from build123d import *

# Parameters (mm, degrees)
CROQUIS1_W              = 163
CROQUIS1_H              = 163
SALIENTE_EXTRUIR1_DEPTH = 3.3
CROQUIS2_R              = 5
SALIENTE_EXTRUIR2_DEPTH = 3
REDONDEO1_R             = 1
CROQUIS3_R              = 3.25
CORTAR_EXTRUIR1_DEPTH   = 3
CROQUIS4_R              = 1.75
CORTAR_EXTRUIR2_DEPTH   = 6.3


with BuildPart() as part:
    # Croquis1 → Saliente-Extruir1 (new body)
    with BuildSketch(Plane(origin=(0, 0, 0), x_dir=(1, 0, 0), z_dir=(0, 1, 0))):
        Rectangle(CROQUIS1_W, CROQUIS1_H)
    extrude(amount=-SALIENTE_EXTRUIR1_DEPTH)

    # Croquis2 → Saliente-Extruir2 (add)
    with BuildSketch(Plane(origin=(0, 0, 0), x_dir=(1, 0, 0), z_dir=(0, 1, 0))):
        with Locations((-75.5, 75.5)):
            Circle(CROQUIS2_R)
        with Locations((75.5, 75.5)):
            Circle(CROQUIS2_R)
        with Locations((-75.5, -75.5)):
            Circle(CROQUIS2_R)
        with Locations((75.5, -75.5)):
            Circle(CROQUIS2_R)
    extrude(amount=SALIENTE_EXTRUIR2_DEPTH)

    # Redondeo1
    redondeo1_edges = [part.edges().sort_by_distance(p)[0] for p in [
        (70.5, 3, -75.5),
        (-80.5, 3, 75.5),
        (70.5, 3, 75.5),
        (-80.5, 3, -75.5),
    ]]
    fillet(redondeo1_edges, radius=REDONDEO1_R)

    # Croquis3 → Cortar-Extruir1 (cut)
    with BuildSketch(Plane.XZ.offset(3.3)):
        with Locations((-75.5, 75.5)):
            Circle(CROQUIS3_R)
        with Locations((75.5, 75.5)):
            Circle(CROQUIS3_R)
        with Locations((-75.5, -75.5)):
            Circle(CROQUIS3_R)
        with Locations((75.5, -75.5)):
            Circle(CROQUIS3_R)
    extrude(amount=-CORTAR_EXTRUIR1_DEPTH, mode=Mode.SUBTRACT)

    # Croquis4 → Cortar-Extruir2 (cut)
    with BuildSketch(Plane(origin=(0, 3, 0), x_dir=(1, 0, 0), z_dir=(0, 1, 0))):
        with Locations((75.5, -75.5)):
            Circle(CROQUIS4_R)
        with Locations((75.5, 75.5)):
            Circle(CROQUIS4_R)
        with Locations((-75.5, 75.5)):
            Circle(CROQUIS4_R)
        with Locations((-75.5, -75.5)):
            Circle(CROQUIS4_R)
    extrude(amount=-CORTAR_EXTRUIR2_DEPTH, mode=Mode.SUBTRACT)


solid = part.part
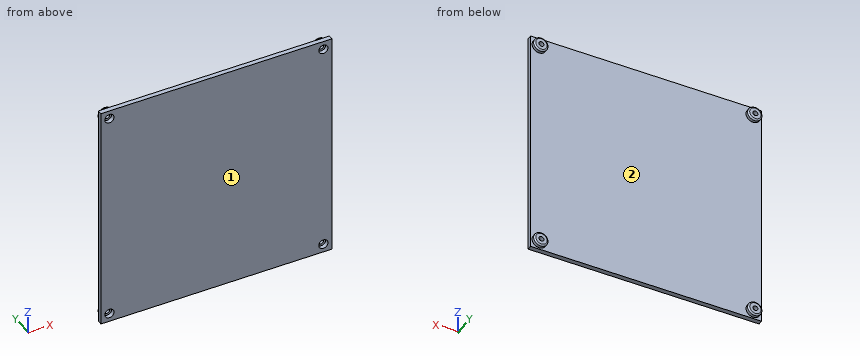
Part model, mm, in its own coordinate system. Face numbers are marked on the shaded views. A direction names the side the tool comes from. Coordinates: 2 decimals unless noted, no trailing zeros. Write each loop counter-clockwise with the first axis right and the second up, starting at its lowest first coordinate (ties: lowest second). Pieces come first, ordered by that corner, then holes. Notation, with made-up numbers: (88, -39) - (133, -39) arc R21 cw to (133, -20) - close; hole circle Ø7 at (35, -6). An arc over 180 degrees is marked (long way). Put each result on its own line as item: value.
1. 3-axis set-ups, long thin cutter, end or side, ignore diameter. For the marked faces 1 and 2: which of +Z, -Z, +X, -X, +Y, -Y reach the whole face in a straight line?
Final values:
face 1: +Z, -Z, +X, -X, -Y
face 2: +Y
2. Band-saw the part on C-C (z = 63). Write the cut outline in (x, y), then the cut area to 3 significant figures.
Final values:
outline: (-81.5, -3.3) - (81.5, -3.3) - (81.5, 0) - (-81.5, 0) - close
area: 538 mm²
3. Flat gauge pins, fed straight in: pin 1 Ø1 at (y, z) = (1.5, 33.5) entering from -X; pin 2 Ø5 at (x, z) = (75.5, -75.5) entering from -Y; pin 3 Ø10 at (x, z) = (-63.5, 4) entering from +Y. Where does each tip first touch, or does it go through?
Final values:
pin 1: passes through
pin 2: stops at y = -0.3
pin 3: stops at y = 0
4. Probe line 1 along Z through (x, y) = (-75.5, 0.5); line 2 along Z through (x, y) = (-75.5, -2.45). List the from-to ranges inside material, lowest first. Write a range as [from, to].
Final values:
line 1: z = [-80.5, -77.25], [-73.75, -70.5], [70.5, 73.75], [77.25, 80.5]
line 2: z = [-81.5, -78.75], [-72.25, 72.25], [78.75, 81.5]
5. Band-saw the part on B-B (x = 66.5). Write the cut outline in (y, z).
Final values:
outline: (-3.3, -81.5) - (0, -81.5) - (0, 81.5) - (-3.3, 81.5) - close
6. Band-saw the part on A-A (y = 1). Write the cut outline in (x, z).
Final values:
outline: circle Ø10 at (-75.5, -75.5); circle Ø10 at (-75.5, 75.5); circle Ø10 at (75.5, -75.5); circle Ø10 at (75.5, 75.5); hole circle Ø3.5 at (-75.5, -75.5); hole circle Ø3.5 at (-75.5, 75.5); hole circle Ø3.5 at (75.5, -75.5); hole circle Ø3.5 at (75.5, 75.5)
